Could you check a few things on this model? Use its own coordinates, in mm. Give positions to 0.01 mm unless a question says otherwise; leave off trailing zeros. Order: outer loops, then holes, each group sorted by start corner. A loop starts at its lowest first (then second) coordinate and runs counter-clockwise, first axis right, second up. Notation, with made-up numbers: (-7, 88.5) -> (49, 88.5) arc R23 cw to (49, 97.5) -> close; hole circle Ø9 at (39.5, 22). An arc over 180 degrees is marked (long way). Use one line per item in the form item = value. Start each with the question number.
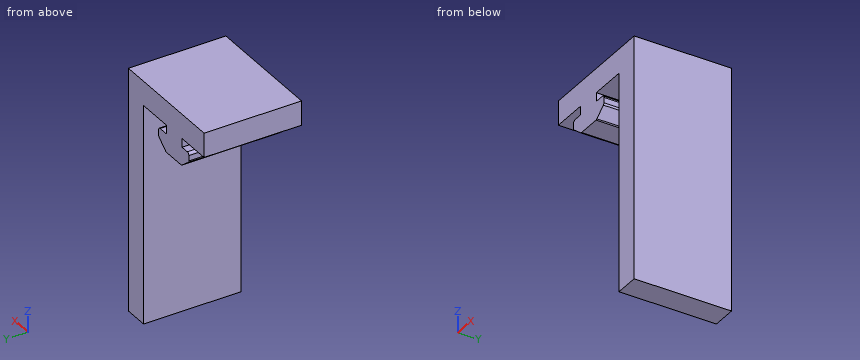
Autodesk Inventor part; units mm, degrees
ref_plane "YZ Plane" through (0, 0, 0) normal (1, 0, 0) x (0, 1, 0)
ref_plane "XZ Plane" through (0, 0, 0) normal (0, 1, 0) x (-1, 0, 0)
ref_plane "XY Plane" through (0, 0, 0) normal (0, 0, 1) x (1, 0, 0)
sketch "Sketch1" plane through (0, 0, 0) normal (0, 1, 0) x (-1, 0, 0)
  line L0 (0, 0) -> (5, 0)
  line L1 (5, -5) -> (5, -50)
  line L2 (5, -50) -> (0, -50)
  line L3 (0, -50) -> (0, 0)
  line L4 (0, 0) -> (25, 0)
  line L5 (25, 0) -> (25, -5)
  line L6 (25, -5) -> (5, -5)
  line L7 (12.5, -5) -> (17.7, -5)
  line L8 (17.7, -5) -> (17.7, -6.8)
  line L9 (17.7, -6.8) -> (12.5, -6.8) construction
  line L10 (12.5, -6.8) -> (12.5, -5)
  line L11 (19.9782, -7.3) -> (19.9782, -8.4084)
  line L12 (19.9782, -8.65) -> (9.9782, -8.65) construction
  line L13 (9.9782, -8.4084) -> (9.9782, -7.3)
  line L14 (17.5282, -8.65) -> (12.4282, -8.65)
  line L15 (12.4282, -8.65) -> (12.4282, -10.5932) construction
  line L16 (12.6024, -10.5932) -> (17.354, -10.5932)
  line L17 (17.5282, -10.5932) -> (17.5282, -8.65) construction
  line L18 (10.1675, -8.8001) -> (12.2917, -10.4849)
  line L19 (19.7889, -8.8001) -> (17.6647, -10.4849)
  line L20 (0, 0) -> (21.2132, -21.2132) construction
  line L21 (0, 0) -> (30, 0) construction
  line L22 (17.6687, -6.6255) -> (12.5, -5) construction
  line L23 (17.7, -5) -> (12.2564, -6.5507) construction
  line L24 (19.9782, -6.8) -> (9.9782, -8.65) construction
  line L25 (19.9782, -8.65) -> (9.9782, -6.8) construction
  line L26 (14.9782, -5.7754) -> (14.9782, -19.5518) construction
  line L27 (17.5282, -8.65) -> (12.4282, -10.5932) construction
  line L28 (12.4282, -8.65) -> (17.5282, -10.5932) construction
  arc A0 (10.4782, -6.8) -> (9.9782, -7.3) centre (10.4782, -7.3) ccw
  arc A1 (9.9782, -8.4084) -> (10.1675, -8.8001) centre (10.4782, -8.4084) ccw
  arc A2 (12.2917, -10.4849) -> (12.6024, -10.5932) centre (12.6024, -10.0932) ccw
  arc A3 (17.354, -10.5932) -> (17.6647, -10.4849) centre (17.354, -10.0932) ccw
  arc A4 (19.7889, -8.8001) -> (19.9782, -8.4084) centre (19.4782, -8.4084) ccw
  arc A5 (19.9782, -7.3) -> (19.4782, -6.8) centre (19.4782, -7.3) ccw
  line L29 (10.4782, -6.8) -> (12.5001, -6.8)
  line L30 (12.5, -6.8) -> (17.7, -6.8) construction
  line L31 (17.7, -6.8) -> (19.4782, -6.8)
  point P0 (17.7, -5)
  point P1 (12.4282, -8.65)
  point P2 (25.5, -11.3)
  point P3 (14.9782, -7.725)
  point P4 (14.9782, -9.6216)
  point P5 (10.0405, -8.65)
  point P6 (19.916, -8.65)
  dimension "d0" = 5
  dimension "d1" = 50
  dimension "d3" = 5
  dimension "d6" = 10
  dimension "d10" = 5.1
  dimension "d11" = 1.9432
  dimension "d13" = 25
  dimension "d14" = 30
  dimension "d15" = 45
  dimension "d18" = 7.5
  dimension "d20" = 0.5
  dimension "d24" = 1.8
  dimension "d25" = 1.85
  dimension "d26" = 5.2
extrude "Extrusion1" add sketch "Sketch1" along normal blind 20
equation "\"d0\" = grosor"
equation "\"d3\" = grosor"
equation "\"d6\" = guia_ancho"
equation "\"d10\" = guia_ancho_menor"
equation "\"d11\" = guia_ancho_menor_espesor"
equation "\"d18\" = guia_sep_borde"
equation "\"d24\" = guia_sep_de_ext"
equation "\"d25\" = guia_ancho_espesor"
equation "\"d26\" = guia_cuello"
equation "\"grosor\" = 5"
equation "\"guia_tol\" = 0.5"
properties part number "Guia_Perfil_test"
(1) Imagine slicing it at D-D (x = -14.5). Write out the boundary of the cut face in (y, z).
(2) Imagine slicing it at C-C (z = -28.5). Write out the boundary of the cut face in (x, y), plus the area to 3 significant figures.
(3) Imagine slicing it at A-A (y = 3.5). Write out the boundary of the cut face in (x, z), plus the area to 3 significant figures.
(4) Please list where these lines run through material, in increasing order: probe 1 along X at (y, z) = (15.75, -8); probe 2 along Z at (x, y) = (-14.25, 18); probe 3 along Z at (x, y) = (-22.5, 6.75).
(5) I'm going to push flat-ended pins straight in: pin 1 Ø1.5 at (x, z) = (-12, -11) entering from +Y; pin 2 Ø8 at (x, y) = (-22, 6.5) entering from -Z; pin 3 Ø0.9 at (y, z) = (5, -5.5) entering from -X; pin 4 Ø12 at (x, y) = (-20, 8.5) entering from -Z. Where does each tip first touch, or does it pass through?
(6) Imagine slicing it at B-B (x = -19). Write out the boundary of the cut face in (y, z).
Calculated:
q1.outline = (0, -10.59) -> (20, -10.59) -> (20, 0) -> (0, 0) -> close
q2.outline = (-5, 0) -> (0, 0) -> (0, 20) -> (-5, 20) -> close
q2.area = 100 mm2
q3.outline = (-25, -5) -> (-17.7, -5) -> (-17.7, -6.8) -> (-19.48, -6.8) arc R0.5 ccw to (-19.98, -7.3) -> (-19.98, -8.41) arc R0.5 ccw to (-19.79, -8.8) -> (-17.66, -10.48) arc R0.5 ccw to (-17.35, -10.59) -> (-12.6, -10.59) arc R0.5 ccw to (-12.29, -10.48) -> (-10.17, -8.8) arc R0.5 ccw to (-9.98, -8.41) -> (-9.98, -7.3) arc R0.5 ccw to (-10.48, -6.8) -> (-12.5, -6.8) -> (-12.5, -5) -> (-5, -5) -> (-5, -50) -> (0, -50) -> (0, 0) -> (-25, 0) -> close
q3.area = 392 mm2
q4.probe_1 = -19.98 to -9.98, -5 to 0
q4.probe_2 = -10.59 to 0
q4.probe_3 = -5 to 0
q5.pin_1 = 20
q5.pin_2 = -10.22
q5.pin_3 = -17.7
q5.pin_4 = -10.59
q6.outline = (0, -9.43) -> (20, -9.43) -> (20, -6.8) -> (0, -6.8) -> close; (0, -5) -> (20, -5) -> (20, 0) -> (0, 0) -> close
